from build123d import *

# Parameters (mm, degrees)
F1_DEPTH = 153.1874
F3_DEPTH = 20.32
F4_R     = 3.1115
F5_DEPTH = 170.688
F7_DEPTH = 153.1884
F8_R     = 15.875
F9_DEPTH = 50.8


with BuildPart() as f1:
    # F0 (on Right) → F1 (new body)
    with BuildSketch(Plane.YZ):
        with BuildLine():
            Line((6.742013631, 7.1882), (-6.742013631, 7.1882))
            ThreePointArc((-6.742013631, 7.1882), (0, -9.8552), (6.742013631, 7.1882))
        make_face()
    extrude(amount=-F1_DEPTH)

    # F2 (on Front) → F3 (cut, symmetric)
    with BuildSketch(Plane.XZ):
        Polygon((-97.2876434091, 9.0090138838), (-123.1138, 9.0090138838), (-123.1138, 0), (-102.489, 0), align=None)
    extrude(amount=F3_DEPTH, both=True, mode=Mode.SUBTRACT)

    # F4 (on face) → F5 (cut)
    with BuildSketch(Plane.YZ):
        Circle(F4_R)
    extrude(amount=-F5_DEPTH, mode=Mode.SUBTRACT)

    # F6 (on face) → F7 (cut, through all)
    with BuildSketch(Plane.YZ):
        with BuildLine():
            Line((-5.969, 4.6482), (-5.969, 7.1882))
            Line((-5.969, 7.1882), (-6.742013631, 7.1882))
            ThreePointArc((-6.742013631, 7.1882), (-7.8199129874, 5.9978269323), (-8.6901785827, 4.6482))
            Line((-8.6901785827, 4.6482), (-5.969, 4.6482))
        make_face()
        with BuildLine():
            Line((5.969, 7.1882), (5.969, 4.6482))
            Line((5.969, 4.6482), (8.6901785827, 4.6482))
            ThreePointArc((8.6901785827, 4.6482), (7.8199129874, 5.9978269323), (6.742013631, 7.1882))
            Line((6.742013631, 7.1882), (5.969, 7.1882))
        make_face()
    extrude(amount=-F7_DEPTH, mode=Mode.SUBTRACT)


with BuildPart() as f9:
    # F8 (on face) → F9 (new body)
    with BuildSketch(Plane.YZ):
        Circle(F8_R)
        with BuildLine():
            Line((5.969, 7.1882), (5.969, 4.6482))
            Line((5.969, 4.6482), (8.6901785827, 4.6482))
            ThreePointArc((8.6901785827, 4.6482), (0, -9.8552), (-8.6901785827, 4.6482))
            Line((-8.6901785827, 4.6482), (-5.969, 4.6482))
            Line((-5.969, 4.6482), (-5.969, 7.1882))
            Line((-5.969, 7.1882), (5.969, 7.1882))
        make_face(mode=Mode.SUBTRACT)
    extrude(amount=F9_DEPTH)


solid = f1.part
Could you check a few things on this model? Use its own coordinates, in mm. A direction names the side the tool comes from. Give positions to 0.01 mm unless a question says otherwise; leave off trailing zeros. Write each loop counter-clockwise with the first axis right and the second up, starting at its lowest first coordinate (ties: lowest second). Pieces come first, ordered by that corner, then holes. Notation, with made-up numbers: (-5, 82.5) - (41, 82.5) arc R20 cw to (41, 106.5) - close; hole circle Ø7 at (32.5, -14.5). An arc over 180 degrees is marked (long way). Use CSV: the item, a comma, the result in double quotes. Start each with the question number.
Item 1: I want a section at A-A, the plane x = -58. Please give me the cut outline in (y, z), then the cut area to 3 significant figures.
Item 2: I'm going to push flat-ended pins straight in: pin 1 (1.5 mm diameter, centred on x = -19.5, z = -1, fed in from +Y); pin 2 (2 mm diameter, centred on x = -144.5, y = -7.5, fed in from +Z); pin 3 (2 mm diameter, centred on x = -72, z = 6.5, fed in from -Y). Where does each tip first touch, or does it pass through?
Item 3: For faces 4 (the face through (-49, 7, 4.648)), 5 (the face through (-113, 6, 0)), 6 (the face through (-138, -7, 4.648)), which set-ups out of +Z, -Z, +X, -X, +Y, -Y let a thin tool reach every point of the face, with its end or its side?
Item 4: If we mould it in two halves opening along X, with no side actions, what happens to faces 1 (the face through (-138, 5.969, 6)), 2 (the face through (-123.114, 0, 4)), 3 (the face through (-153.187, 2, -3))? For each: pulls with the +X half, pulls with the -X half, needs draft (parallel to the pull), parting line crosses it, or undercut.
Item 5: I want a section at B-B, the plane y = 0. Please give me the cut outline in (x, z), then the cut area to 3 significant figures.
Item 6: If I drill on line 1 along Z through (x, y) = (-67.5, 0); line 2 along Y through (x, z) = (-82, 0); line 3 along Z through (x, y) = (-113.5, 0), over which ranges is the centre line in solid material (lowest first)?
Findings:
1,outline,"(-8.69, 4.65) arc R9.86 ccw (long way) to (8.69, 4.65) - (5.97, 4.65) - (5.97, 7.19) - (-5.97, 7.19) - (-5.97, 4.65) - close; hole circle Ø6.22 at (0, 0)"
1,area,"241 mm2"
2,pin 1,"stops at y = 9.85"
2,pin 2,"stops at z = 4.65"
2,pin 3,"stops at y = -5.97"
3,face 4,"+Z, +X, -X, +Y"
3,face 5,"+Z, +Y, -Y"
3,face 6,"+Z, +X, -X, -Y"
4,face 1,"needs draft"
4,face 2,"undercut"
4,face 3,"pulls with the -X half"
5,outline,"(-153.19, -9.86) - (0, -9.86) - (0, -3.11) - (-153.19, -3.11) - close; (-153.19, 3.11) - (-123.11, 3.11) - (-123.11, 7.19) - (-153.19, 7.19) - close; (-100.69, 3.11) - (0, 3.11) - (0, 7.19) - (-98.34, 7.19) - close"
5,area,"1,560 mm2"
6,line 1,"z = -9.86 to -3.11, 3.11 to 7.19"
6,line 2,"y = -9.86 to -3.11, 3.11 to 9.86"
6,line 3,"z = -9.86 to -3.11"
